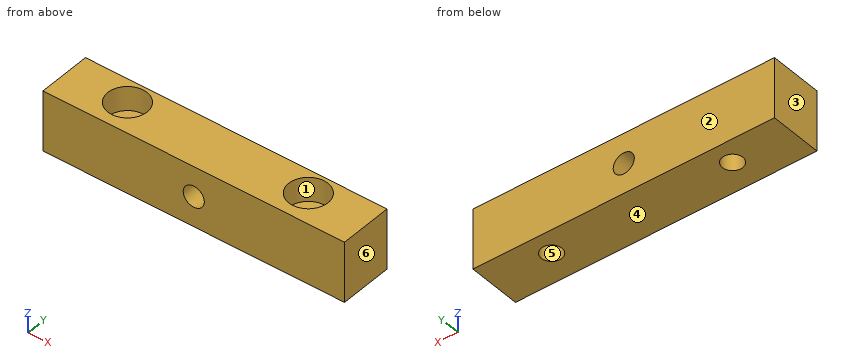
```python
from build123d import *

# Parameters (mm, degrees)
F0_W           = 50
F0_H           = 10
F1_DEPTH       = 10
F3_D           = 3.4
F3_CBORE_D     = 6.5
F3_CBORE_DEPTH = 4
F5_D           = 3.5
F6_DEPTH       = 1.2


with BuildPart() as f1:
    # F0 (on Front) → F1 (new body)
    with BuildSketch(Plane.XZ):
        with Locations((-13.0036683753, -0.9258947149)):
            Rectangle(F0_W, F0_H)
    extrude(amount=F1_DEPTH)

    # F3 (through all)
    with Locations(Plane.XY.offset(4.0741052851)):
        with Locations((-28.0036683753, -5), (1.9963316247, -5)):
            CounterBoreHole(F3_D / 2, F3_CBORE_D / 2, F3_CBORE_DEPTH)

    # F5 (through all)
    with Locations(Plane.XZ.offset(10)):
        with Locations((-13.0036683753, -0.9258947149)):
            Hole(F5_D / 2)

    # F6 (cut): a face of the model
    f6_faces = [f1.faces().sort_by_distance(p)[0] for p in [
        (-13.0036683753, 0, 3.5642033337),
    ]]
    extrude(f6_faces, amount=-F6_DEPTH, mode=Mode.SUBTRACT)


solid = f1.part
```
Here's how the part is built. I have some questions about the finished solid (model axes, mm). Face numbers are marked on the shaded views. A direction names the side the tool comes from. Give positions to 0.01 mm unless a question says otherwise; leave off trailing zeros. Loops run counter-clockwise (first coordinate to the right, second up) from the corner with the lowest first, then second, coordinate; pieces in that order, holes last. Notation, with made-up numbers: (19, -7.5) -> (69, -7.5) arc R21 cw to (69, 10.5) -> close; hole circle Ø3 at (-8.75, 29). An arc over 180 degrees is marked (long way). Use one line per item in the form item = value. Start each with the question number.
1) Imagine slicing it at C-C (x = -25.5). Please give me the cut outline in (y, z).
2) Imagine slicing it at D-D (z = 3.25). Please give me the cut outline in (x, y).
3) Please list where these lines run through material, in increasing order: line 1 along X through (y, z) = (-5.5, 1.25); line 2 along Z through (x, y) = (-26, -5); line 3 along X through (y, z) = (-6.75, 1.25).
4) Imagine slicing it at A-A (z = -2). Please give me the cut outline in (x, y).
5) Thinking about a two-plate mould opening in X: for the marked faces 3, 4, 5 and 6, which applies, +X half, -X half, draft (parallel to the pull), parting line (faces both ways), or undercut?
6) For P1, Ø5, axis at x = -28, y = -5, coming from the +Z side, with a flat end and sliding along its axis, tell me the tip position at first contact or that it passes through.
7) Imagine slicing it at B-B (y = -5). Please give me the cut outline in (x, z).
8) Which directions (+Z, -Z, +X, -X, +Y, -Y) give clear straight access to the entire face, cutting with the end or side of a thin tool? Please do the marked faces 1 and 2.
Check values:
q1.outline = (-10, -5.93) -> (-1.2, -5.93) -> (-1.2, 4.07) -> (-2.93, 4.07) -> (-2.93, 0.07) -> (-7.07, 0.07) -> (-7.07, 4.07) -> (-10, 4.07) -> close
q2.outline = (-38, -10) -> (12, -10) -> (12, -1.2) -> (-38, -1.2) -> close; hole circle Ø6.5 at (-28, -5); hole circle Ø6.5 at (2, -5)
q3.line_1 = -38 to -31.21, -24.79 to -1.21, 5.21 to 12
q3.line_2 = -5.93 to 0.07
q3.line_3 = -38 to -30.74, -25.27 to -0.74, 4.73 to 12
q4.outline = (-38, -10) -> (-14.39, -10) -> (-14.39, -1.2) -> (-38, -1.2) -> close; (-11.62, -10) -> (12, -10) -> (12, -1.2) -> (-11.62, -1.2) -> close; hole circle Ø3.4 at (-28, -5); hole circle Ø3.4 at (2, -5)
q5.face_3 = -X half
q5.face_4 = draft
q5.face_5 = undercut
q5.face_6 = +X half
q6.P1 = 0.07
q7.outline = (-38, -5.93) -> (-29.7, -5.93) -> (-29.7, 0.07) -> (-31.25, 0.07) -> (-31.25, 4.07) -> (-38, 4.07) -> close; (-26.3, -5.93) -> (0.3, -5.93) -> (0.3, 0.07) -> (-1.25, 0.07) -> (-1.25, 4.07) -> (-24.75, 4.07) -> (-24.75, 0.07) -> (-26.3, 0.07) -> close; (3.7, -5.93) -> (12, -5.93) -> (12, 4.07) -> (5.25, 4.07) -> (5.25, 0.07) -> (3.7, 0.07) -> close; hole circle Ø3.5 at (-13, -0.93)
q8.face_1 = +Z
q8.face_2 = +Z, -Z, +X, -X, +Y
